CAD build for the part. Positions are in the model's coordinates, mm. A direction names the side the tool comes from. Round coordinates to 2 decimals unless told otherwise and drop trailing zeros. Loops run counter-clockwise (first coordinate to the right, second up) from the corner with the lowest first, then second, coordinate; pieces in that order, holes last.
from build123d import *

# Parameters (mm, degrees)
F0_R      = 30
F0_R_2    = 15
F1_DEPTH  = 18
F2_W      = 20
F2_H      = 33
F3_DEPTH  = 16.5
F5_DEPTH  = 45
F9_DEPTH  = 45.001
F10_DEPTH = 45.001
F11_R     = 6
F12_R     = 13.2790561914
F13_DEPTH = 20
F14_R     = 10


with BuildPart() as f1:
    # F0 (on Front) → F1 (new body, symmetric)
    with BuildSketch(Plane.XZ):
        Circle(F0_R)
        Circle(F0_R_2, mode=Mode.SUBTRACT)
    extrude(amount=F1_DEPTH, both=True)

    # F2 (on Front) → F3 (join, symmetric)
    with BuildSketch(Plane.XZ):
        with Locations((35, 0)):
            Rectangle(F2_W, F2_H)
    extrude(amount=F3_DEPTH, both=True)

    # F4 (on face) → F5 (join)
    with BuildSketch(Plane.YZ.offset(45)):
        Polygon((-16.5, 9.5262794416), (-16.5, -9.5262794416), (0, -19.0525588833), (16.5, -9.5262794416), (16.5, 9.5262794416), (0, 19.0525588833), align=None)
    extrude(amount=F5_DEPTH)

    # F7 (on mid) → F8 (revolve, cut)
    with BuildSketch(Plane(origin=(0, 0, 0), x_dir=(-1, 0, 0), z_dir=(0, 1, 0))):
        Polygon((-90, 19.0525588833), (-90, 13.2790561914), (-80, 19.0525588833), align=None)
    revolve(axis=Axis((76.7741315067, 0, 0), (1, 0, 0)), mode=Mode.SUBTRACT)

    # F9 (cut, through all): a face of the model
    f9_faces = [f1.faces().sort_by_distance(p)[0] for p in [
        (45, 0, 17.3508529611),
    ]]
    extrude(f9_faces, amount=-F9_DEPTH, mode=Mode.SUBTRACT)

    # F10 (cut, through all): a face of the model
    f10_faces = [f1.faces().sort_by_distance(p)[0] for p in [
        (45, 0, -17.3508529611),
    ]]
    extrude(f10_faces, amount=-F10_DEPTH, mode=Mode.SUBTRACT)

    # F11
    f11_edges = [f1.edges().sort_by_distance(p)[0] for p in [
        (45, -10.460581, -13.01314),
        (45, -10.460581, 13.01314),
        (45, 10.460581, 13.01314),
        (45, 10.460581, -13.01314),
    ]]
    fillet(f11_edges, radius=F11_R)

    # F12 (on face) → F13 (join)
    with BuildSketch(Plane.YZ.offset(90)):
        Circle(F12_R)
    extrude(amount=F13_DEPTH)

    # F14
    f14_edges = [f1.edges().sort_by_distance(p)[0] for p in [
        (25.05494, 0, 16.5),
        (25.05494, 0, -16.5),
    ]]
    fillet(f14_edges, radius=F14_R)


solid = f1.part
Item 1: 3-axis set-ups, long thin cutter, end or side, ignore diameter. For faces 4 (the flat face through (51, 0, 16.5)), 5 (the flat face through (67.48, 10.55, 12.96)), 6 (the flat face through (67.48, -10.55, -12.96)), 7 (the flat face through (67.48, 10.38, -13.06)), 8 (the flat face through (67.48, -10.38, 13.06)): which of +Z, -Z, +X, -X, +Y, -Y reach the whole face in a straight line?
Verdict:
face 4: +Z, +X, +Y, -Y
face 5: +Z, +X, +Y
face 6: -Z, +X, -Y
face 7: -Z, +X, +Y
face 8: +Z, +X, -Y
Item 2: Cut at A-A (y = 0). List the corners of the cut face in (x, z) (3 decimals).
Verdict:
outline: (22.472, -19.875) arc R10 cw to (29.962, -16.5) - (84.421, -16.5) - (90, -13.279) - (110, -13.279) - (110, 13.279) - (90, 13.279) - (84.421, 16.5) - (29.962, 16.5) arc R10 cw to (22.472, 19.875) arc R30 ccw (long way) to start; hole circle Ø30 at (0, 0)
Item 3: Mould opens along X. For faces 1 (the flat face through (110, 0, 0)), 2 (the cylindrical face through (-14.985, 0.252, 0.66)), 3 (the flat face through (53, -16.5, 0)) say: released by +X, released by -X, zero draft, split by the parting line, or undercut.
Verdict:
face 1: released by +X
face 2: undercut
face 3: zero draft
Item 4: Cut at B-B (z = 0). List the corners of the cut face in (x, y).
Verdict:
outline: (-30, -18) - (-15, -18) - (-15, 18) - (-30, 18) - close; (15, -18) - (30, -18) - (30, -16.5) - (84.42, -16.5) - (90, -13.28) - (110, -13.28) - (110, 13.28) - (90, 13.28) - (84.42, 16.5) - (30, 16.5) - (30, 18) - (15, 18) - close
Item 5: Flat gauge pins, fed straight in: P1, Ø1.5, axis at y = -12.5, z = 12.5, coming from the +X side; P2, Ø6, axis at x = -13, y = 3, coming from the +Z side; P3, Ø8, axis at y = -13.5, z = -23.5, coming from the +X side. Where does each tip first touch, or does it go through?
Verdict:
P1: stops at x = 83.68
P2: stops at z = 28.28
P3: stops at x = 22.82
Item 6: Cut at D-D (x = 63). List the corners of the cut face in (y, z), plus the area to 3 significant figures.
Verdict:
outline: (-16.5, -9.53) - (-4.42, -16.5) - (4.42, -16.5) - (16.5, -9.53) - (16.5, 9.53) - (4.42, 16.5) - (-4.42, 16.5) - (-16.5, 9.53) - close
area: 921 mm2
Item 7: Wall check: L1, parallel to Z at x = 0, y = -4; L2, parallel to X at y = -12.5, z = 10; L3, parallel to Z at x = -6.5, y = -16. Give the ranges that are in metal, low to high.
Verdict:
L1: z = -30 to -15, 15 to 30
L2: x = -28.28 to -11.18, 11.18 to 85.27
L3: z = -29.29 to -13.52, 13.52 to 29.29
Item 8: Cut at C-C (x = 9.5). List the corners of the cut face in (y, z), plus the area to 3 significant figures.
Verdict:
outline: (-18, -28.46) - (18, -28.46) - (18, -11.61) - (-18, -11.61) - close; (-18, 11.61) - (18, 11.61) - (18, 28.46) - (-18, 28.46) - close
area: 1,210 mm2
